Verification items for the finished model (mm, model axes). Coordinates: 2 decimals unless noted, no trailing zeros. Order: outer loops, then holes, each group sorted by start corner. A loop starts at its lowest first (then second) coordinate and runs counter-clockwise, first axis right, second up. Notation, with made-up numbers: (-7.5, -34.5) -> (18.5, -34.5) arc R20 cw to (18.5, 0.5) -> close; hole circle Ø8 at (-38, 87.5). An arc over 180 degrees is marked (long way). Write each question's results on one line, items separated by ' | '. Start each with the question number.
(1) Cross-section at A-A on y = -20. Enter the section's corners in (x, z).
(2) Draft check along Z on faces 1 (the cylindrical face through (-15, 32, 0)), 2 (the flat face through (-14, -8, 0)), 3 (the cylindrical face through (-15.52, 5.95, 18.22)). Enter one of: +Z half, -Z half, draft (parallel to the pull), parting line (faces both ways), or undercut.
(3) Cross-section at D-D on y = 0. Enter the section's corners in (x, z).
(4) Thickness scan on probe 1 along Z at (x, y) = (-16.2, -9.5); probe 2 along Z at (x, y) = (-15.2, -11); probe 3 along Y at (x, z) = (-15.15, 18). Record the ranges inside material, lowest first. Write a range as [from, to].
(5) Cross-section at C-C on y = -7. Enter the section's corners in (x, z), and give its area (3 significant figures).
(6) Cross-section at B-B on z = 0. Enter the section's corners in (x, y).
```python
from build123d import *

# Parameters (mm, degrees)
AXIAL_BLANK_PROFILE_W                     = 3
AXIAL_BLANK_PROFILE_H                     = 32
MAGNET_BASE_START                         = -17
MAGNET_BASE_LOCATOR_BORES_SKETCH_R        = 6.15
MAGNET_BASE_LOCATOR_BORES_SKETCH_R_2      = 4.15
MAGNET_BASE_LOCATOR_BORES_DEPTH           = 3
OPEN_START                                = -17
OPEN_FITTING_ROUTE_RELIEFS_SKETCH_R       = 8.25
OPEN_FITTING_ROUTE_RELIEFS_DEPTH          = 3
THREE_START                               = -17
THREE_M2_LOCATOR_CLEARANCE_HOLES_SKETCH_R = 1.2
THREE_M2_LOCATOR_CLEARANCE_HOLES_DEPTH    = 3


with BuildPart() as part:
    # Axial blank profile → Native revolved blank (revolve)
    with BuildSketch(Plane.XY, mode=Mode.PRIVATE) as native_revolved_blank_sk:
        with Locations((-15.5, 16)):
            Rectangle(AXIAL_BLANK_PROFILE_W, AXIAL_BLANK_PROFILE_H)
    revolve(native_revolved_blank_sk.sketch.rotate(Axis((-60, 0, 0), (1, 0, 0)), 90), axis=Axis((-60, 0, 0), (1, 0, 0)))

    # Magnet-base locator bores sketch → Magnet-base locator bores (cut)
    with BuildSketch(Plane(origin=(0, 0, 0), x_dir=(0, 0, -1), z_dir=(1, 0, 0)).offset(MAGNET_BASE_START)):
        Circle(MAGNET_BASE_LOCATOR_BORES_SKETCH_R)
        with Locations((0, 20)):
            Circle(MAGNET_BASE_LOCATOR_BORES_SKETCH_R_2)
        with Locations((-17.320508076, 10)):
            Circle(MAGNET_BASE_LOCATOR_BORES_SKETCH_R_2)
        with Locations((-17.320508076, -10)):
            Circle(MAGNET_BASE_LOCATOR_BORES_SKETCH_R_2)
        with Locations((0, -20)):
            Circle(MAGNET_BASE_LOCATOR_BORES_SKETCH_R_2)
        with Locations((17.320508076, -10)):
            Circle(MAGNET_BASE_LOCATOR_BORES_SKETCH_R_2)
        with Locations((17.320508076, 10)):
            Circle(MAGNET_BASE_LOCATOR_BORES_SKETCH_R_2)
    extrude(amount=MAGNET_BASE_LOCATOR_BORES_DEPTH, mode=Mode.SUBTRACT)

    # Open fitting-route reliefs sketch → Open fitting-route reliefs (cut)
    with BuildSketch(Plane(origin=(0, 0, 0), x_dir=(0, 0, -1), z_dir=(1, 0, 0)).offset(OPEN_START)):
        with Locations((-13, 22.516660498)):
            Circle(OPEN_FITTING_ROUTE_RELIEFS_SKETCH_R)
        with Locations((13, 22.516660498)):
            Circle(OPEN_FITTING_ROUTE_RELIEFS_SKETCH_R)
    extrude(amount=OPEN_FITTING_ROUTE_RELIEFS_DEPTH, mode=Mode.SUBTRACT)

    # Three M2 locator clearance holes sketch → Three M2 locator clearance holes (cut)
    with BuildSketch(Plane(origin=(0, 0, 0), x_dir=(0, 0, -1), z_dir=(1, 0, 0)).offset(THREE_START)):
        with Locations((-24.248711306, 14)):
            Circle(THREE_M2_LOCATOR_CLEARANCE_HOLES_SKETCH_R)
        with Locations((0, -28)):
            Circle(THREE_M2_LOCATOR_CLEARANCE_HOLES_SKETCH_R)
        with Locations((24.248711306, 14)):
            Circle(THREE_M2_LOCATOR_CLEARANCE_HOLES_SKETCH_R)
    extrude(amount=THREE_M2_LOCATOR_CLEARANCE_HOLES_DEPTH, mode=Mode.SUBTRACT)


solid = part.part
```
Results are:
1) outline: (-17, -24.98) -> (-14, -24.98) -> (-14, -4.15) -> (-17, -4.15) -> close; (-17, 4.15) -> (-14, 4.15) -> (-14, 24.98) -> (-17, 24.98) -> close
2) face 1: parting line | face 2: draft | face 3: undercut
3) outline: (-17, -32) -> (-14, -32) -> (-14, -6.15) -> (-17, -6.15) -> close; (-17, 6.15) -> (-14, 6.15) -> (-14, 32) -> (-17, 32) -> close
4) probe 1: z = [-30.56, -21.44], [-13.2, 13.2], [21.44, 30.56] | probe 2: z = [-30.05, -21.35], [-13.29, 13.29], [21.35, 30.05] | probe 3: y = [-26.46, -14.09], [-5.91, 5.91], [14.09, 15.95]
5) outline: (-17, -31.22) -> (-14, -31.22) -> (-14, -20.19) -> (-17, -20.19) -> close; (-17, -14.45) -> (-14, -14.45) -> (-14, 14.45) -> (-17, 14.45) -> close; (-17, 20.19) -> (-14, 20.19) -> (-14, 31.22) -> (-17, 31.22) -> close | area: 153 mm2
6) outline: (-17, -32) -> (-14, -32) -> (-14, -29.2) -> (-17, -29.2) -> close; (-17, -26.8) -> (-14, -26.8) -> (-14, -24.15) -> (-17, -24.15) -> close; (-17, -15.85) -> (-14, -15.85) -> (-14, -6.15) -> (-17, -6.15) -> close; (-17, 6.15) -> (-14, 6.15) -> (-14, 15.85) -> (-17, 15.85) -> close; (-17, 24.15) -> (-14, 24.15) -> (-14, 32) -> (-17, 32) -> close
